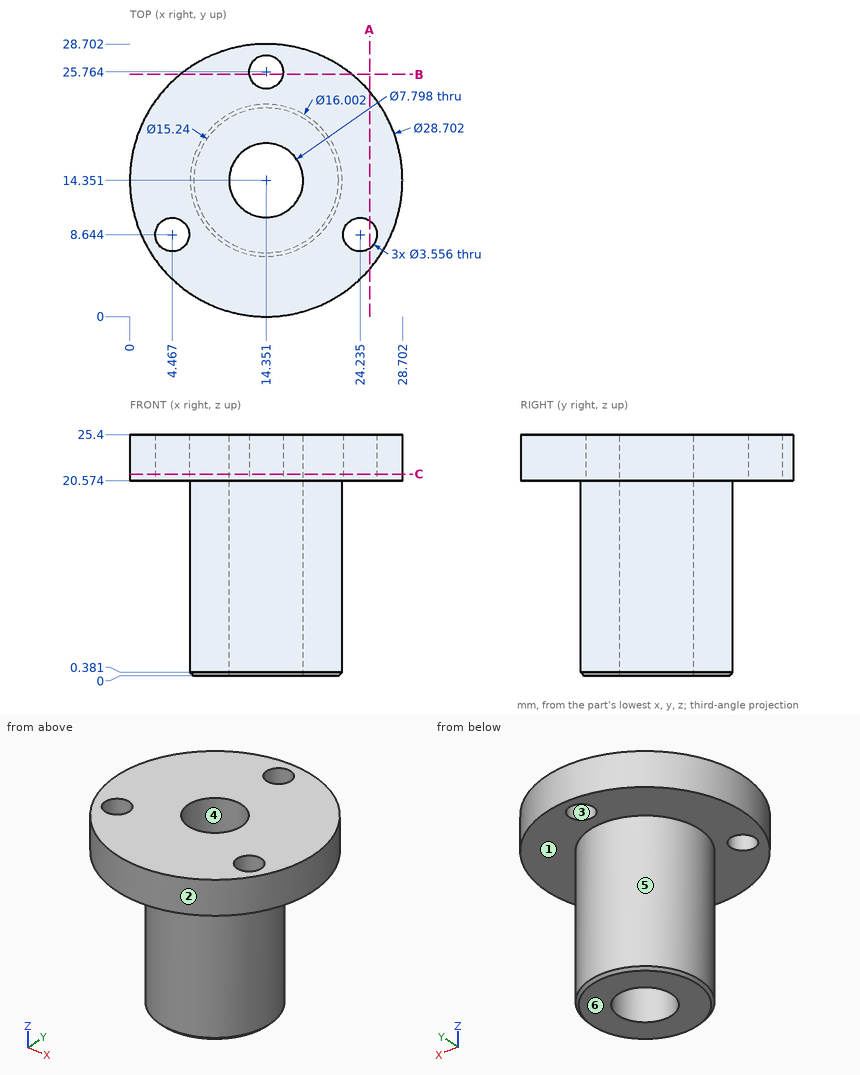
Design review of the part shown in the three views and the two pictorial views. Dimensions are in mm from the part's minimum x, y and z. A direction names the side the tool comes from. Round coordinates to 2 decimals unless told otherwise and drop trailing zeros. Loops run counter-clockwise (first coordinate to the right, second up) from the corner with the lowest first, then second, coordinate; pieces in that order, holes last. Notation, with made-up numbers: M -12.75,-14.75 L 2.25,-14.75 A21 ccw 2.25,0.25 Z; hole C 33,-29.5 d9. An arc over 180 degrees is marked long. Answer as a JSON object with one key per item and string values.
Item 1: We need section C-C, the plane z = 21.25. State how many separate pieces and enclosed holes the cut face has.
Check sheet entries:
{"separate pieces": "1", "enclosed holes": "4"}
Item 2: We need section B-B, the plane y = 25.5. State the section outline as (x, z) points (1 decimal).
Check sheet entries:
{"outline": "M 5.3,20.6 L 12.6,20.6 L 12.6,25.4 L 5.3,25.4 Z; M 16.1,20.6 L 23.4,20.6 L 23.4,25.4 L 16.1,25.4 Z"}
Item 3: Clearance check with flat-ended pins moving along their axes: P1, Ø2, axis at y = 3.5, z = 20, coming from the -X side; P2, Ø1, axis at x = 11, z = 15.5, coming from the -Y side (1 decimal); P3, Ø10, axis at x = 14.351, y = 14.351, coming from the +Z side; P4, Ø2, axis at y = 18.5, z = 11, coming from the -X side (1 decimal). State where each tip first meets the part, or that it passes through.
Check sheet entries:
{"P1": "x = 4.09", "P2": "y = 6.9", "P3": "z = 25.4", "P4": "x = 7"}
Item 4: For line 1 along X through (y, z) = (15, 24) (1 decimal); line 2 along Y through (x, z) = (14.75, 11); line 3 along Y through (x, z) = (13, 20.25) (1 decimal), list the stretches that pass through material, from the lowest coordinate up.
Check sheet entries:
{"line 1": "0 to 10.5, 18.2 to 28.7", "line 2": "6.36 to 10.47, 18.23 to 22.34", "line 3": "6.5 to 10.7, 18 to 22.2"}
Item 5: Tool access review of the marked faces 5 and 6: name each direction out of +Z, -Z, +X, -X, +Y, -Y from which nothing blocks a thin tool from reaching the whole face with its end or side.
Check sheet entries:
{"face 5": "-Z", "face 6": "-Z, +X, -X, +Y, -Y"}
Item 6: The part is to be moulded in two halves that separate along Y. For the marked faces 1, 2, 3 and 4, say which applies: +Y half, -Y half, draft (parallel to the pull), parting line (faces both ways), or undercut.
Check sheet entries:
{"face 1": "draft", "face 2": "parting line", "face 3": "undercut", "face 4": "undercut"}
Item 7: We need section A-A, the plane x = 25.25. State the section outline as (y, z) points (1 decimal).
Check sheet entries:
{"outline": "M 5,20.6 L 7.2,20.6 L 7.2,25.4 L 5,25.4 Z; M 10.1,20.6 L 23.7,20.6 L 23.7,25.4 L 10.1,25.4 Z"}
